Verification items for the finished model (mm, model axes). Face numbers are marked on the shaded views. A direction names the side the tool comes from. Give positions to 0.01 mm unless a question says otherwise; leave off trailing zeros. Write each loop counter-clockwise with the first axis right and the second up, starting at its lowest first coordinate (ties: lowest second). Pieces come first, ordered by that corner, then holes. Notation, with made-up numbers: M -9,0 L 1,0 A23 ccw 1,12 Z; hole C -7,35 d10. An arc over 180 degrees is marked long. Answer as a JSON object with one key per item and string values.
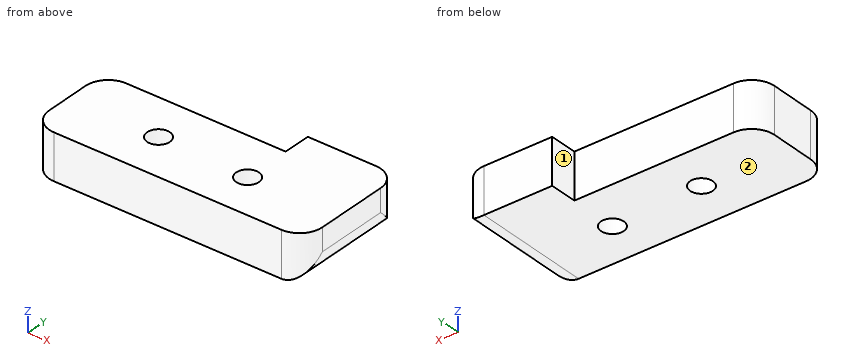
```python
from build123d import *

# Parameters (mm, degrees)
F1_DEPTH = 25.4
F2_R     = 12.7
F4_D     = 12.7


with BuildPart() as f1:
    # F0 (on Top) → F1 (new body)
    with BuildSketch(Plane.XY):
        Polygon((-0.620216, 50.796214), (0, 0), (152.388641, 1.860649), (151.768425, 68.068433), (100.972211, 67.448217), (100.972211, 52.036646), align=None)
    extrude(amount=F1_DEPTH)

    # F2
    f2_edges = [f1.edges().sort_by_distance(p)[0] for p in [
        (-0.620216, 50.796214, 12.7),
        (152.078533, 34.964541, 0),
        (152.388641, 1.860649, 12.7),
        (0, 0, 12.7),
        (151.768425, 68.068433, 12.7),
    ]]
    fillet(f2_edges, radius=F2_R)

    # F4 (through all)
    with Locations(Plane.XY.offset(25.4)):
        with Locations((101.289892, 25.398107), (50.489892, 26.098501)):
            Hole(F4_D / 2)


solid = f1.part
```
1) Go/stop test with flat-tipped pins: pin 1 (8 mm diameter, centred on x = 123.5, z = 7, fed in from -Y); pin 2 (1 mm diameter, centred on x = 45, z = 12, fed in from +Y); pin 3 (6 mm diameter, centred on x = 47, y = 29.5, fed in from +Z); pin 4 (4 mm diameter, centred on x = 118, z = 21.5, fed in from -Y). Record where each tip stops, or that it passes through.
Completed:
{"pin 1": "stops at y = 1.46", "pin 2": "stops at y = 51.36", "pin 3": "stops at z = 25.4", "pin 4": "stops at y = 1.42"}
2) Section check B-B on x = 59.5. Record the boundary of the cut face in (y, z), and give its area (3 significant figures).
Completed:
{"outline": "M 0.73,0 L 51.53,0 L 51.53,25.4 L 0.73,25.4 Z", "area": "1,290 mm2"}
3) Access from +Z, -Z, +X, -X, +Y, -Y to the whole of each face (thin tool, end or side, straight path). Record for the marked faces 1 and 2.
Completed:
{"face 1": "+Z, -Z, -X, +Y", "face 2": "-Z, +X, -X, +Y, -Y"}
4) Section check A-A on z = 9.5. Record the boundary of the cut face in (x, y).
Completed:
{"outline": "M -0.47,38.1 L -0.16,12.7 A12.7 ccw 12.7,0.16 L 139.73,1.71 A12.7 ccw 151.89,11.32 L 151.45,58.53 A12.7 ccw 139.03,67.91 L 100.97,67.45 L 100.97,52.04 L 12.08,50.95 A12.7 ccw Z; hole C 50.49,26.1 d12.7; hole C 101.29,25.4 d12.7"}
5) Thickness scan on L1, parallel to X at y = 25, z = 21.25; L2, parallel to X at y = 25, z = 2.75; L3, parallel to Y at x = 140.5, z = 11.25. Record the ranges inside material, lowest first.
Completed:
{"L1": "x = -0.31 to 44.24, 56.74 to 94.95, 107.63 to 152.17", "L2": "x = -0.31 to 44.24, 56.74 to 94.95, 107.63 to 147.36", "L3": "y = 1.74 to 67.85"}
6) Section check C-C on z = 17.5. Record the boundary of the cut face in (x, y), and give its area (3 significant figures).
Completed:
{"outline": "M -0.47,38.1 L -0.16,12.7 A12.7 ccw 12.7,0.16 L 139.73,1.71 A12.7 ccw 152.27,14.52 L 151.89,55.33 A12.7 ccw 139.03,67.91 L 100.97,67.45 L 100.97,52.04 L 12.08,50.95 A12.7 ccw Z; hole C 50.49,26.1 d12.7; hole C 101.29,25.4 d12.7", "area": "8,140 mm2"}
7) Section check D-D on y = 30. Count the separate pieces of the cut face and the enclosed holes in it, and give its area (3 significant figures).
Completed:
{"separate pieces": "3", "enclosed holes": "0", "area": "3,360 mm2"}
